Work out the finished part from the listing and answer in its coordinate system (mm). Face numbers are marked on the shaded views. A direction names the side the tool comes from. Coordinates: 2 decimals unless noted, no trailing zeros. Loops run counter-clockwise (first coordinate to the right, second up) from the corner with the lowest first, then second, coordinate; pieces in that order, holes last. Notation, with made-up numbers: M 22,38.5 L 34,38.5 A27 ccw 34,71.5 Z; hole C 23.5,35 d10. An arc over 180 degrees is marked long. Write each question's results on one line, items separated by ' | '.
```python
from build123d import *

# Parameters (mm, degrees)
F0_W     = 770
F0_H     = 1470
F1_DEPTH = 390
F2_W     = 330
F2_H     = 330
F3_DEPTH = 390


with BuildPart() as f1:
    # F0 (on Front) → F1 (new body)
    with BuildSketch(Plane.XZ):
        with Locations((385, 735)):
            Rectangle(F0_W, F0_H)
    extrude(amount=-F1_DEPTH)

    # F2 (on face) → F3 (cut, through all)
    with BuildSketch(Plane.XZ):
        with Locations((212.5, 562.5)):
            Rectangle(F2_W, F2_H)
        with Locations((557.5, 562.5)):
            Rectangle(F2_W, F2_H)
        with Locations((557.5, 907.5)):
            Rectangle(F2_W, F2_H)
        with Locations((212.5, 907.5)):
            Rectangle(F2_W, F2_H)
        with Locations((212.5, 1252.5)):
            Rectangle(F2_W, F2_H)
        with Locations((557.5, 1252.5)):
            Rectangle(F2_W, F2_H)
        with Locations((212.5, 217.5)):
            Rectangle(F2_W, F2_H)
        with Locations((557.5, 217.5)):
            Rectangle(F2_W, F2_H)
    extrude(amount=-F3_DEPTH, mode=Mode.SUBTRACT)


solid = f1.part
```
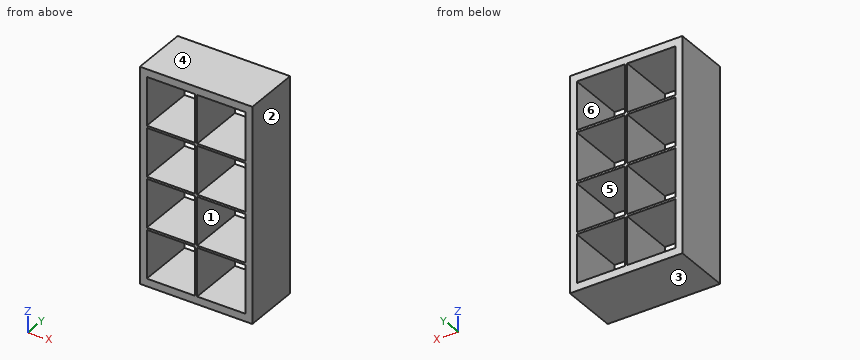
1) Find section B-B, the plane z = 596. Give the vertices of the cut face in (x, y).
Check result:
outline: M 0,0 L 47.5,0 L 47.5,390 L 0,390 Z; M 377.5,0 L 392.5,0 L 392.5,390 L 377.5,390 Z; M 722.5,0 L 770,0 L 770,390 L 722.5,390 Z
2) Find section C-C, the plane y = 113.5. Give the number of separate pieces and of enclosed holes in the cut face, and give its area (3 significant figures).
Check result:
separate pieces: 1 | enclosed holes: 8 | area: 261,000 mm^2
3) Which of the six approach directions +Z, -Z, +X, -X, +Y, -Y give full straight-line access (tool end or side, diameter ignored) to the marked faces 1 and 2?
Check result:
face 1: +Y, -Y | face 2: +Z, -Z, +X, +Y, -Y
4) Find section A-A, the plane x = 617. Give the vertices of the cut face in (y, z), and give its area (3 significant figures).
Check result:
outline: M 0,0 L 390,0 L 390,52.5 L 0,52.5 Z; M 0,382.5 L 390,382.5 L 390,397.5 L 0,397.5 Z; M 0,727.5 L 390,727.5 L 390,742.5 L 0,742.5 Z; M 0,1072.5 L 390,1072.5 L 390,1087.5 L 0,1087.5 Z; M 0,1417.5 L 390,1417.5 L 390,1470 L 0,1470 Z | area: 58,500 mm^2
5) For a pull along Z with two mould halves and no side action, classify the marked faces 3, 4, 5 and 6 as released by +Z, released by -Z, zero draft, split by the parting line, or undercut.
Check result:
face 3: released by -Z | face 4: released by +Z | face 5: undercut | face 6: undercut
6) Straight lines are drawn through the part: probe 1 along Z at (x, y) = (86.5, 286.5); probe 2 along X at (y, z) = (216.5, 1132.5). For each, find the intervals that lie inside material, in ascending order. Write a range as [from, to].
Check result:
probe 1: [0, 52.5], [382.5, 397.5], [727.5, 742.5], [1072.5, 1087.5], [1417.5, 1470] | probe 2: [0, 47.5], [377.5, 392.5], [722.5, 770]
